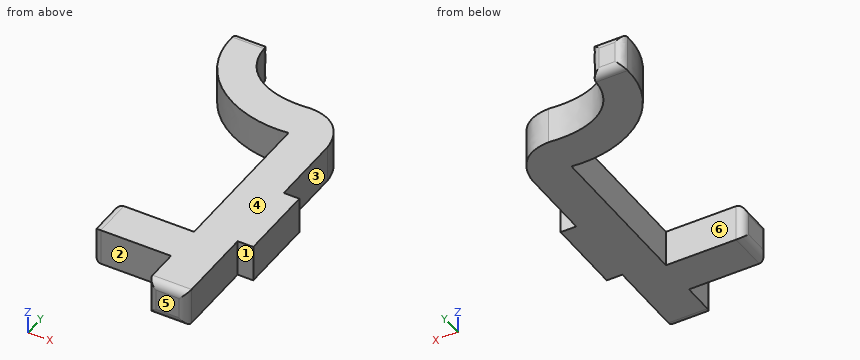
```python
from build123d import *

# Parameters (mm, degrees)
F0_W     = 2
F0_H     = 10
F1_DEPTH = 4.7
F2_R     = 1
F3_R     = 1
F4_R     = 1


with BuildPart() as f1:
    # F0 (on Top) → F1 (new body)
    with BuildSketch(Plane.XY):
        with BuildLine():
            Line((-9.963439, 33.065276), (-13.963439, 33.065276))
            add(Edge.make_bspline(
                [(-13.963439, 33.065276), (-14.933051, 24.878523), (-7.296724, 19.661296), (0, 20.5)],
                knots=[0, 0, 0, 0, 18.784669, 18.784669, 18.784669, 18.784669], degree=3))
            Line((0, 20.5), (0, 0))
            Line((0, 0), (-10, 0))
            Line((-10, 0), (-10, -5))
            Line((-10, -5), (0, -5))
            Line((0, -5), (0, -10))
            Line((0, -10), (5, -10))
            Line((5, -10), (5, 1))
            Line((5, 1), (5, 11))
            Line((5, 11), (5, 20.5))
            add(Edge.make_bspline(
                [(0, 25.5), (4.53556, 25.319498), (4.944229, 21.235214), (5, 20.5)],
                knots=[0, 0, 0, 0, 7.071068, 7.071068, 7.071068, 7.071068], degree=3))
            add(Edge.make_bspline(
                [(-9.963439, 33.065276), (-10.31617, 28.009873), (-6.350763, 24.845181), (0, 25.5)],
                knots=[0, 0, 0, 0, 12.510137, 12.510137, 12.510137, 12.510137], degree=3))
        make_face()
        with Locations((6, 6)):
            Rectangle(F0_W, F0_H)
    extrude(amount=F1_DEPTH)

    # F2
    f2_edges = [f1.edges().sort_by_distance(p)[0] for p in [
        (-9.963439, 33.065276, 2.35),
        (-13.963439, 33.065276, 2.35),
        (-11.963439, 33.065276, 0),
        (-11.963439, 33.065276, 4.7),
    ]]
    fillet(f2_edges, radius=F2_R)

    # F3
    f3_edges = [f1.edges().sort_by_distance(p)[0] for p in [
        (-10, 0, 2.35),
        (-10, -5, 2.35),
        (-10, -2.5, 0),
        (-10, -2.5, 4.7),
    ]]
    fillet(f3_edges, radius=F3_R)

    # F4
    f4_edges = [f1.edges().sort_by_distance(p)[0] for p in [
        (0, -10, 2.35),
        (5, -10, 2.35),
        (2.5, -10, 0),
        (2.5, -10, 4.7),
    ]]
    fillet(f4_edges, radius=F4_R)


solid = f1.part
```
Check sheet for the modelled part. Datum: model origin and axes. Units: mm. Face numbers are marked on the shaded views. A direction names the side the tool comes from. Coordinates: 2 decimals unless noted, no trailing zeros. Write each loop counter-clockwise with the first axis right and the second up, starting at its lowest first coordinate (ties: lowest second). Pieces come first, ordered by that corner, then holes. Notation, with made-up numbers: (8.25, -37.5) - (32.25, -37.5) arc R13 cw to (32.25, -25.5) - close; hole circle Ø5 at (64.5, 27.5). An arc over 180 degrees is marked (long way). One line per question, with ' | ' between items.
Item 1: Sectioned sample at B-B on y = 20. Record the boundary of the cut face in (x, z).
Determined:
outline: (0, 0) - (5, 0) - (5, 4.7) - (0, 4.7) - close
Item 2: Gauge pin test, flat ends, axial feed: P1, Ø8, axis at x = -10, y = 1.5, coming from the +Z side; P2, Ø2, axis at x = 5.5, z = 3, coming from the -Y side; P3, Ø1, axis at x = 0.5, z = 4, coming from the +Y side; P4, Ø0.6, axis at x = 6.5, z = 3, coming from the +Y side. Record the tip position at first contact, or that the pin passes through.
Determined:
P1: stops at z = 4.7 | P2: stops at y = -9.87 | P3: stops at y = 25.5 | P4: stops at y = 11
Item 3: Mould release check, pull along Y, two halves, no side actions. Record for the marked faces 4, 5 and 6: pulls with the +Y half, pulls with the -Y half, needs draft (parallel to the pull), parting line crosses it, or undercut.
Determined:
face 4: needs draft | face 5: pulls with the -Y half | face 6: undercut
Item 4: Access from +Z, -Z, +X, -X, +Y, -Y to the whole of each face (thin tool, end or side, straight path). Record for the marked faces 1, 2 and 3.
Determined:
face 1: +Z, -Z, +X, -Y | face 2: +Z, -Z, -X, -Y | face 3: +Z, -Z, +X, +Y
Item 5: Sectioned sample at A-A on y = 3.5. Record the boundary of the cut face in (x, z).
Determined:
outline: (0, 0) - (7, 0) - (7, 4.7) - (0, 4.7) - close
Item 6: Thickness scan on line 1 (X direction, y = 8, z = 2.5); line 2 (X direction, y = 19.5, z = 3.45); line 3 (Y direction, x = -0.75, z = 2.7). Record the ranges inside material, lowest first. Write a range as [from, to].
Determined:
line 1: x = [0, 7] | line 2: x = [0, 5] | line 3: y = [-5, 0], [20.44, 25.44]
